Work out the finished part from the listing and answer in its coordinate system (mm). A direction names the side the tool comes from. Give positions to 0.01 mm unless a question says otherwise; leave off trailing zeros. Loops run counter-clockwise (first coordinate to the right, second up) from the corner with the lowest first, then second, coordinate; pieces in that order, holes last. Notation, with made-up numbers: (-20.75, 21.5) - (29.25, 21.5) arc R17 cw to (29.25, 41.5) - close; hole circle Ø11 at (60, 25.25). An arc over 180 degrees is marked (long way). One line per question, with ' | ' between items.
from build123d import *

# Parameters (mm, degrees)
SKETCH1_R           = 7.5
BOSS_EXTRUDE1_DEPTH = 7
SKETCH2_R           = 1.5
BOSS_EXTRUDE2_DEPTH = 15
SKETCH3_W           = 5
SKETCH3_H           = 3.05
CUT_EXTRUDE1_DEPTH  = 6
SKETCH4_R           = 7.5
BOSS_EXTRUDE3_DEPTH = 7


with BuildPart() as part:
    # Sketch1 → Boss-Extrude1 (new body)
    with BuildSketch(Plane(origin=(0, 0, 0), x_dir=(1, 0, 0), z_dir=(0, 1, 0))):
        Circle(SKETCH1_R)
    extrude(amount=BOSS_EXTRUDE1_DEPTH)

    # Sketch2 → Boss-Extrude2 (add)
    with BuildSketch(Plane(origin=(0, 7, 0), x_dir=(1, 0, 0), z_dir=(0, 1, 0))):
        Circle(SKETCH2_R)
    extrude(amount=BOSS_EXTRUDE2_DEPTH)

    # Sketch3 → Cut-Extrude1 (cut)
    with BuildSketch(Plane.XZ):
        Rectangle(SKETCH3_W, SKETCH3_H)
    extrude(amount=-CUT_EXTRUDE1_DEPTH, mode=Mode.SUBTRACT)

    # Sketch4 → Boss-Extrude3 (add)
    with BuildSketch(Plane(origin=(0, 22, 0), x_dir=(1, 0, 0), z_dir=(0, 1, 0))):
        Circle(SKETCH4_R)
    extrude(amount=BOSS_EXTRUDE3_DEPTH)


solid = part.part
1. Find section D-D on z = 0. Write down the section's boundary in (x, y), then the cut area to 3 significant figures.
Evaluation:
outline: (-7.5, 0) - (-2.5, 0) - (-2.5, 6) - (2.5, 6) - (2.5, 0) - (7.5, 0) - (7.5, 7) - (1.5, 7) - (1.5, 22) - (7.5, 22) - (7.5, 29) - (-7.5, 29) - (-7.5, 22) - (-1.5, 22) - (-1.5, 7) - (-7.5, 7) - close | area: 225 mm2
2. Determine the mould class of faces 4 (the cylindrical face through (-7.493, 25.451, -0.33)), 5 (the flat face through (2, 7, 0)), 6 (the flat face through (0, 3, -1.525)), 7 (the flat face through (-2.5, 3, 0)) for opening direction X: +X half, -X half, draft (parallel to the pull), parting line (faces both ways), or undercut.
Evaluation:
face 4: parting line | face 5: draft | face 6: undercut | face 7: undercut
3. Flat-ended cylindrical pins translate along their axes: pin 1 (1 mm diameter, centred on y = 8, z = -3, fed in from -X); pin 2 (1 mm diameter, centred on y = 16.5, z = -0.5, fed in from +X). Find the tip coordinate at first contact, or state that the pin passes through.
Evaluation:
pin 1: through | pin 2: x = 1.5
4. Which of the six approach directions +Z, -Z, +X, -X, +Y, -Y give full straight-line access (tool end or side, diameter ignored) to faces 1 (the cylindrical face through (-1.5, 14.4, -0.07)), 2 (the flat face through (0, 0, 2)), 3 (the flat face through (0, 6, 0))?
Evaluation:
face 1: none | face 2: +Z, -Z, +X, -X, -Y | face 3: -Y
5. Consider L1, parallel to Y at x = -5.5, z = -4.5; L2, parallel to Z at x = 0, y = 14.75. Determine where each line is inside the solid, lowest interval first.
Evaluation:
L1: 0 to 7, 22 to 29 | L2: -1.5 to 1.5
6. Find section C-C on x = 0. Write down the section's boundary in (y, z) (3 decimals).
Evaluation:
outline: (0, -7.5) - (7, -7.5) - (7, -1.5) - (22, -1.5) - (22, -7.5) - (29, -7.5) - (29, 7.5) - (22, 7.5) - (22, 1.5) - (7, 1.5) - (7, 7.5) - (0, 7.5) - (0, 1.525) - (6, 1.525) - (6, -1.525) - (0, -1.525) - close
7. Find section B-B on z = 3. Write down the section's boundary in (x, y).
Evaluation:
outline: (-6.87, 0) - (6.87, 0) - (6.87, 7) - (-6.87, 7) - close; (-6.87, 22) - (6.87, 22) - (6.87, 29) - (-6.87, 29) - close
8. Find section A-A on x = 6. Write down the section's boundary in (y, z).
Evaluation:
outline: (0, -4.5) - (7, -4.5) - (7, 4.5) - (0, 4.5) - close; (22, -4.5) - (29, -4.5) - (29, 4.5) - (22, 4.5) - close
